Answer from the drawing. Dimensions are ordinates in mm from the lowest x, y and z of the part. A direction names the side the tool comes from. Give positions to 0.01 mm unless a question says otherwise; leave off trailing zeros. Order: outer loops, then holes, each group sorted by start corner. A loop starts at its lowest first (then second) coordinate and runs counter-clockwise, first axis right, second up. Notation, with made-up numbers: (-13, -19) - (45, -19) arc R31 ccw to (45, 11) - close; hole circle Ø4 at (-36.75, -18). An arc over 180 degrees is marked (long way). One line per item, written item: value. Start each with the question number.
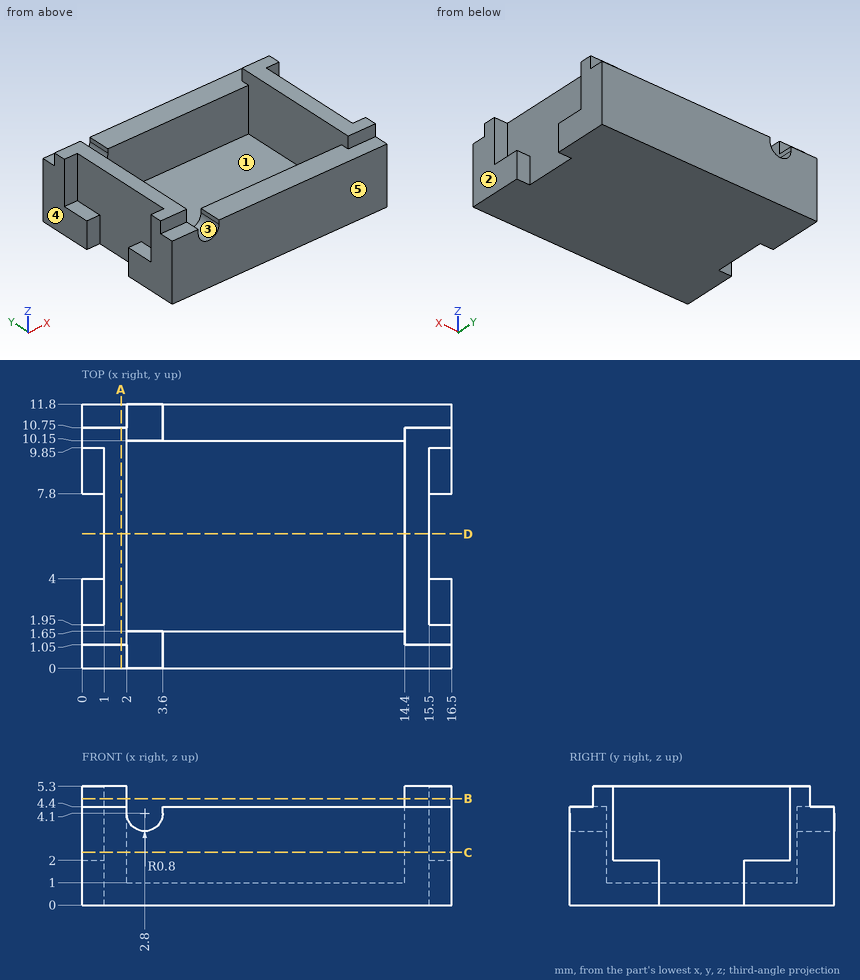
1) Section A-A on x = 1.75 is taken. Write down the section's boundary in (y, z).
2) Section D-D on y = 6 is taken. Write down the section's boundary in (x, z).
3) Section C-C on z = 2.35 is taken. Write down the section's boundary in (x, y), plus the area to 3 significant figures.
4) Each of these flat-tipped pins is pushed along its axis until it touches: pin 1 (4 mm diameter, centred on x = 6, y = 5.5, fed in from +Z); pin 2 (0.5 mm diameter, centred on x = 16, y = 3, fed in from +Z); pin 3 (0.5 mm diameter, centred on x = 1, z = 5, fed in from +Y). Where does it stop, or does it pass through?
5) For the marked faces 1 and 2, determine the directions among +Z, -Z, +X, -X, +Y, -Y from which every point of the face is accessible in a straight line to the end or side of a thin tool.
6) Section B-B on z = 4.75 is taken. Write down the section's boundary in (x, y), plus the area to 3 significant figures.
7) The mould has two halves that part along X. Classify the marked faces 3, 4 and 5: +X half, -X half, draft (parallel to the pull), parting line (faces both ways), or undercut.
8) Find the intervals of material crossed by probe 1 along X at (y, z) = (8, 2.1); probe 2 along Y at (x, z) = (6.5, 3.65); probe 3 along X at (y, z) = (10, 5.05), in increasing order. Write a range as from..to.
Solved:
1. outline: (0, 0) - (11.8, 0) - (11.8, 4.4) - (10.75, 4.4) - (10.75, 5.3) - (1.05, 5.3) - (1.05, 4.4) - (0, 4.4) - close
2. outline: (1, 0) - (15.5, 0) - (15.5, 5.3) - (14.4, 5.3) - (14.4, 1) - (2, 1) - (2, 5.3) - (1, 5.3) - close
3. outline: (0, 0) - (16.5, 0) - (16.5, 1.95) - (15.5, 1.95) - (15.5, 9.85) - (16.5, 9.85) - (16.5, 11.8) - (0, 11.8) - (0, 9.85) - (1, 9.85) - (1, 1.95) - (0, 1.95) - close; hole (2, 1.65) - (14.4, 1.65) - (14.4, 10.15) - (2, 10.15) - close
3. area: 73.5 mm2
4. pin 1: stops at z = 1
4. pin 2: stops at z = 2
4. pin 3: stops at y = 10.75
5. face 1: +Z
5. face 2: +Z, -Z, +X, +Y, -Y
6. outline: (0, 1.05) - (2, 1.05) - (2, 10.75) - (0, 10.75) - (0, 9.85) - (1, 9.85) - (1, 1.95) - (0, 1.95) - close; (14.4, 1.05) - (16.5, 1.05) - (16.5, 1.95) - (15.5, 1.95) - (15.5, 9.85) - (16.5, 9.85) - (16.5, 10.75) - (14.4, 10.75) - close
6. area: 24.0 mm2
7. face 3: undercut
7. face 4: -X half
7. face 5: draft
8. probe 1: x = 1..2, 14.4..15.5
8. probe 2: y = 0..1.65, 10.15..11.8
8. probe 3: x = 0..2, 14.4..16.5
